```python
from build123d import *

# Parameters (mm, degrees)
SKETCH_1_R          = 55
EXTRUDE_1_DEPTH     = 2
SKETCH_2_R          = 1.65
CUT_EXTRUDE_1_DEPTH = 2
SKETCH_2_4_R        = 1.65
CUT_EXTRUDE_3_DEPTH = 2
SKETCH_3_R          = 1.5
CUT_EXTRUDE_4_DEPTH = 10


with BuildPart() as part:
    # 草图1 → 凸台-拉伸1 (new body)
    with BuildSketch(Plane(origin=(0, 0, 0), x_dir=(1, 0, 0), z_dir=(0, 1, 0))):
        Circle(SKETCH_1_R)
    extrude(amount=EXTRUDE_1_DEPTH)

    # 草图2 → 切除-拉伸1 (cut)
    with BuildSketch(Plane(origin=(0, 2, 0), x_dir=(1, 0, 0), z_dir=(0, 1, 0))):
        with Locations((36.016872787, -33.590882314)):
            Circle(SKETCH_2_R)
    extrude(amount=-CUT_EXTRUDE_1_DEPTH, mode=Mode.SUBTRACT)

    # 草图2<4> → 切除-拉伸3 (cut)
    with BuildSketch(Plane(origin=(0, 2, 0), x_dir=(1, 0, 0), z_dir=(0, 1, 0))):
        with Locations((-36.016872787, 33.590882314)):
            Circle(SKETCH_2_4_R)
        with Locations((33.590882314, 36.016872787)):
            Circle(SKETCH_2_4_R)
        with Locations((-33.590882314, -36.016872787)):
            Circle(SKETCH_2_4_R)
    extrude(amount=-CUT_EXTRUDE_3_DEPTH, mode=Mode.SUBTRACT)

    # 草图3 → 切除-拉伸4 (cut)
    with BuildSketch(Plane(origin=(0, 2, 0), x_dir=(1, 0, 0), z_dir=(0, 1, 0))):
        with Locations((-26.846179952, -21.454198237)):
            Circle(SKETCH_3_R)
        with Locations((-19.533109335, -28.274681956)):
            Circle(SKETCH_3_R)
        with Locations((5.892141898, 13.648540723)):
            Circle(SKETCH_3_R)
        with Locations((13.205212514, 6.828057004)):
            Circle(SKETCH_3_R)
        Polygon((-28.822223675, -15.509011007), (-0.176192057, 15.205885583), (15.181256238, 0.882869774), (-13.46477538, -29.832026816), align=None)
    extrude(amount=-CUT_EXTRUDE_4_DEPTH, mode=Mode.SUBTRACT)


solid = part.part
```
Verification items for the finished model (mm, model axes). A direction names the side the tool comes from. Coordinates: 2 decimals unless noted, no trailing zeros. Write each loop counter-clockwise with the first axis right and the second up, starting at its lowest first coordinate (ties: lowest second). Pieces come first, ordered by that corner, then holes. Notation, with made-up numbers: M 83.25,39 L 95.25,39 A29 cw 95.25,70 Z; hole C 88.5,87.25 d9. An arc over 180 degrees is marked long. Answer as a JSON object with one key per item and string values. Group by question number.
(1) Cross-section at B-B, the plane z = 10. Record the cut outline in (x, y), and give its area (3 significant figures).
(2) Release check for a two-part mould opening along X. For faces 3 (the face through (11, 2, 11)), 4 (the face through (-11.923, 0.986, 53.692)), 5 (the face through (32.375, 1.014, -37.132)) record: +X half, -X half, draft (parallel to the pull), parting line (faces both ways), or undercut.
(3) Cross-section at D-D, the plane z = 44. Record the cut outline in (x, y).
(4) Material ranges on line 1 (Z direction, x = 12, y = 0.3); line 2 (Z direction, x = 9, y = 1.2); line 3 (Z direction, x = -33, y = 0.5), recorded low to high.
(5) Gauge pin test, flat end, axial feed: pin 1 (2.5 mm diameter, centred on x = 33.59, z = -36.02, fed in from -Y). Record the tip position at first contact, or that the pin passes through.
(6) Cross-section at A-A, the plane y = 1.25. State how many separate pieces and enclosed holes the cut face has, and give its area (3 significant figures).
(7) Cross-section at C-C, the plane x = 10. Record the cut outline in (y, z), and give its area (3 significant figures).
(8) Tool access check on faces 1 (the face through (11, 0, 11)), 2 (the face through (-14.7, 1.014, 0.367)). Record the directions out of +Z, -Z, +X, -X, +Y, -Y that give a thin tool (end or side, any length) a straight path to the whole face; none if there is none.
Reply:
{
 "1": {"outline": "M -54.08,0 L -23.68,0 L -23.68,2 L -54.08,2 Z; M 5.03,0 L 54.08,0 L 54.08,2 L 5.03,2 Z", "area": "159 mm²"},
 "2": {"face 3": "draft", "face 4": "parting line", "face 5": "undercut"},
 "3": {"outline": "M -33,0 L 33,0 L 33,2 L -33,2 Z"},
 "4": {"line 1": "-53.67 to -7.72, -5.94 to -3.85, 2.53 to 53.67", "line 2": "-54.26 to -6.65, 5.74 to 54.26", "line 3": "-44 to 34.48, 37.56 to 44"},
 "5": {"pin 1": "through"},
 "6": {"separate pieces": "1", "enclosed holes": "9", "area": "8,560 mm²"},
 "7": {"outline": "M 0,-54.08 L 2,-54.08 L 2,-5.72 L 0,-5.72 Z; M 0,4.67 L 2,4.67 L 2,54.08 L 0,54.08 Z", "area": "196 mm²"},
 "8": {"face 1": "+Z, -Z, +X, -X, -Y", "face 2": "+Y, -Y"}
}
